Input: part model. Units: mm. Frame: model coordinates. Face numbers are marked on the shaded views. A direction names the side the tool comes from. Coordinates: 2 decimals unless noted, no trailing zeros. Order: outer loops, then holes, each group sorted by start corner. A loop starts at its lowest first (then second) coordinate and runs counter-clockwise, first axis right, second up. Notation, with made-up numbers: M -26.5,51.5 L 2.5,51.5 A26 ccw 2.5,68.5 Z; hole C 51,31.25 d8. An arc over 180 degrees is marked long. One line per item, written item: value.
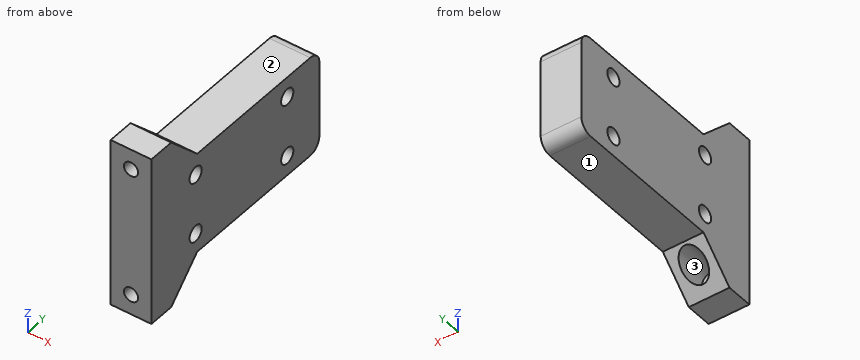
```python
from build123d import *

# Parameters (mm, degrees)
SKETCH1_W           = 10
SKETCH1_H           = 42
BOSS_EXTRUDE1_DEPTH = 3
SKETCH7_W           = 10
SKETCH7_H           = 25
BOSS_EXTRUDE4_DEPTH = 52
CHAMFER2_SIZE       = 12
SKETCH8_R           = 1.75
CUT_EXTRUDE1_DEPTH  = 60.084684987
SKETCH9_R           = 3
CUT_EXTRUDE2_DEPTH  = 50
FILLET1_R           = 3
SKETCH10_R          = 2
CUT_EXTRUDE3_DEPTH  = 60.715994507


with BuildPart() as part:
    # Sketch1 → Boss-Extrude1 (new body)
    with BuildSketch(Plane(origin=(0, 0, 0), x_dir=(1, 0, 0), z_dir=(0, 1, 0))):
        Rectangle(SKETCH1_W, SKETCH1_H)
    extrude(amount=BOSS_EXTRUDE1_DEPTH)

    # Sketch7 → Boss-Extrude4 (add)
    with BuildSketch(Plane(origin=(0, 3, 0), x_dir=(1, 0, 0), z_dir=(0, 1, 0))):
        Rectangle(SKETCH7_W, SKETCH7_H)
    extrude(amount=BOSS_EXTRUDE4_DEPTH)

    # Chamfer2
    # the kernel refuses this chamfer: 12 mm, written as the material it adds along each edge
    with BuildSketch(Plane(origin=(5, 3, 12.5), x_dir=(0, -0.02749587661058638, 0.9996219169112968), z_dir=(-1, 0, 0))) as chamfer2_piece_1_section:
        Polygon((CHAMFER2_SIZE * 0.999621916911, CHAMFER2_SIZE * 0.0274958766106), (-CHAMFER2_SIZE * 0.0274958766106, CHAMFER2_SIZE * 0.999621916911), (0, 0), align=None)
    chamfer2_piece_1 = extrude(amount=10, mode=Mode.PRIVATE)
    chamfer2_piece_1 = split(chamfer2_piece_1, bisect_by=Plane(origin=(0, 7.292994705, 21), z_dir=(0, 0, -1)), keep=Keep.TOP, mode=Mode.PRIVATE)
    add(chamfer2_piece_1)
    with BuildSketch(Plane(origin=(-5, 3, -12.5), x_dir=(0, -0.02749587661058638, -0.9996219169112968), z_dir=(1, 0, 0))) as chamfer2_piece_2_section:
        Polygon((CHAMFER2_SIZE * 0.999621916911, CHAMFER2_SIZE * 0.0274958766106), (-CHAMFER2_SIZE * 0.0274958766106, CHAMFER2_SIZE * 0.999621916911), (0, 0), align=None)
    chamfer2_piece_2 = extrude(amount=10, mode=Mode.PRIVATE)
    chamfer2_piece_2 = split(chamfer2_piece_2, bisect_by=Plane(origin=(0, 7.292994705, -21), z_dir=(0, 0, 1)), keep=Keep.TOP, mode=Mode.PRIVATE)
    add(chamfer2_piece_2)

    # Sketch8 → Cut-Extrude1 (cut, through all)
    with BuildSketch(Plane(origin=(0, 55, 0), x_dir=(1, 0, 0), z_dir=(0, 1, 0))):
        with Locations(Location((0, 16, 0), (0, 0, 270))):
            Circle(SKETCH8_R)
        with Locations(Location((0, -16, 0), (0, 0, 270))):
            Circle(SKETCH8_R)
    extrude(amount=-CUT_EXTRUDE1_DEPTH, mode=Mode.SUBTRACT)

    # Sketch9 → Cut-Extrude2 (cut)
    with BuildSketch(Plane(origin=(0, 55, 0), x_dir=(1, 0, 0), z_dir=(0, 1, 0))):
        with Locations(Location((0, 16, 0), (0, 0, 270))):
            Circle(SKETCH9_R)
        with Locations(Location((0, -16, 0), (0, 0, 270))):
            Circle(SKETCH9_R)
    extrude(amount=-CUT_EXTRUDE2_DEPTH, mode=Mode.SUBTRACT)

    # Fillet1
    fillet1_edges = [part.edges().sort_by_distance(p)[0] for p in [
        (0, 55, -12.5),
        (0, 55, 12.5),
    ]]
    fillet(fillet1_edges, radius=FILLET1_R)

    # Sketch10 → Cut-Extrude3 (cut, through all)
    with BuildSketch(Plane.ZY.offset(5)):
        with Locations((-7.5, 14.5)):
            Circle(SKETCH10_R)
        with Locations((7.5, 14.5)):
            Circle(SKETCH10_R)
        with Locations((-7.5, 44.5)):
            Circle(SKETCH10_R)
        with Locations((7.5, 44.5)):
            Circle(SKETCH10_R)
    extrude(amount=-CUT_EXTRUDE3_DEPTH, mode=Mode.SUBTRACT)


solid = part.part
```
(1) Cut plane B-B on z = -16. Output: boundary loops of the cut face in (x, y).
Data:
outline: M -5,0 L -1.75,0 L -1.75,5 L -3,5 L -3,11.5 L -5,11.5 Z; M 1.75,0 L 5,0 L 5,11.5 L 3,11.5 L 3,5 L 1.75,5 Z
(2) Cut plane C-C on z = 7.5. Output: boundary loops of the cut face in (x, y), plus the area to 3 significant figures.
Data:
outline: M -5,0 L 5,0 L 5,12.5 L -5,12.5 Z; M -5,16.5 L 5,16.5 L 5,42.5 L -5,42.5 Z; M -5,46.5 L 5,46.5 L 5,55 L -5,55 Z
area: 470 mm2
(3) Ray query, line 1 (Y direction, x = 1.5, z = 7); line 2 (X direction, y = 2.4, z = 16); line 3 (Y direction, x = 1.5, z = -7.5). Return the intervals inside material, ascending. Write a range as from..to.
Data:
line 1: y = 0..12.56, 16.44..42.56, 46.44..55
line 2: x = -5..-1.75, 1.75..5
line 3: y = 0..12.5, 16.5..42.5, 46.5..55
(4) Cut plane A-A on x = 0. Give the number of separate pieces and of enclosed holes in the cut face, plus the area to 3 significant figures.
Data:
separate pieces: 3
enclosed holes: 4
area: 1,390 mm2
(5) Cut plane D-D on y = 44.5. Output: boundary loops of the cut face in (x, z).
Data:
outline: M -5,-12.5 L 5,-12.5 L 5,-9.5 L -5,-9.5 Z; M -5,-5.5 L 5,-5.5 L 5,5.5 L -5,5.5 Z; M -5,9.5 L 5,9.5 L 5,12.5 L -5,12.5 Z
(6) Access query for the marked faces 1, 2 and 3. Directions: +Z, -Z, +X, -X, +Y, -Y. A direction counts if a zero-diameter tool reaches every point of the face in a straight line with its end or side. Return the directions, or none.
Data:
face 1: -Z, +X, -X, +Y
face 2: +Z, +X, -X, +Y
face 3: +Y
(7) First-contact query: pin 1 (6 mm diameter, centred on x = -0.5, y = 40, fed in from +Z); pin 2 (3 mm diameter, centred on x = -2.5, y = 37.5, fed in from -Z); pin 3 (4.5 mm diameter, centred on x = 0, z = -16, fed in from +Y). Flat tips, straight axial feed; report the tip coordinate or a pass-through.
Data:
pin 1: stops at z = 12.5
pin 2: stops at z = -12.5
pin 3: stops at y = 5
